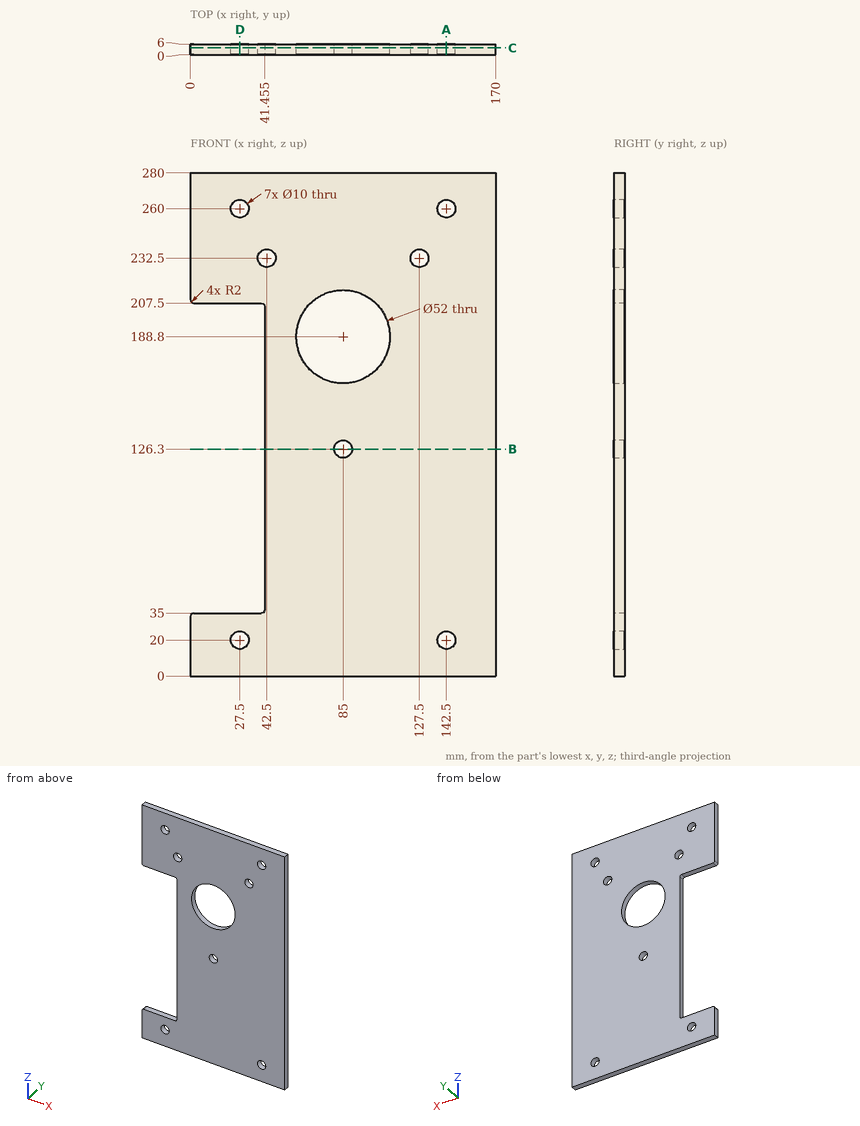
Geometry: see drawing. Coordinates: mm, zero at the bounding-box minimum. Give positions to 0.01 mm unless a question says otherwise; leave off trailing zeros. Write each loop counter-clockwise with the first axis right and the second up, starting at its lowest first coordinate (ties: lowest second). Pieces come first, ordered by that corner, then holes. Notation, with made-up numbers: M 72,76.25 L 122,76.25 A21 ccw 122,99.25 Z; hole C 56,-38.75 d3. An arc over 180 degrees is marked long. Answer as a JSON object with one key per item and string values.
Q1. Cut plane D-D, the plane x = 27.5. Return the cut outline in (y, z).
Geometry check:
{"outline": "M 0,0 L 6,0 L 6,15 L 0,15 Z; M 0,25 L 6,25 L 6,35 L 0,35 Z; M 0,207.5 L 6,207.5 L 6,255 L 0,255 Z; M 0,265 L 6,265 L 6,280 L 0,280 Z"}
Q2. Cut plane B-B, the plane z = 126.3. Return the cut outline in (x, y) (1 decimal), then the cut area to 3 significant figures.
Geometry check:
{"outline": "M 41.5,0 L 80,0 L 80,6 L 41.5,6 Z; M 90,0 L 170,0 L 170,6 L 90,6 Z", "area": "711 mm^2"}
Q3. Contact query for a flat-ended pin moving along its axis: P1, Ø1.5, axis at y = 2.5, z = 117.5, coming from the -X side (1 decimal). Output: stop coordinate, or through.
Geometry check:
{"P1": "stops at x = 41.5"}
Q4. Cut plane C-C, the plane y = 3.85. Count the separate pieces of the cut face and the enclosed holes in it, then the cut area to 3 significant figures.
Geometry check:
{"separate pieces": "1", "enclosed holes": "8", "area": "37,800 mm^2"}
Q5. Cut plane A-A, the plane x = 142.5. Return the cut outline in (y, z).
Geometry check:
{"outline": "M 0,0 L 6,0 L 6,15 L 0,15 Z; M 0,25 L 6,25 L 6,255 L 0,255 Z; M 0,265 L 6,265 L 6,280 L 0,280 Z"}
Q6. Ray query, line 1 along X through (y, z) = (2.65, 232.5); line 2 along Z through (x, y) = (142.5, 3.7); line 3 along X through (y, z) = (2.55, 126.3) (1 decimal). Return the intervals inside material, ascending.
Geometry check:
{"line 1": "x = 0 to 37.5, 47.5 to 122.5, 132.5 to 170", "line 2": "z = 0 to 15, 25 to 255, 265 to 280", "line 3": "x = 41.5 to 80, 90 to 170"}
